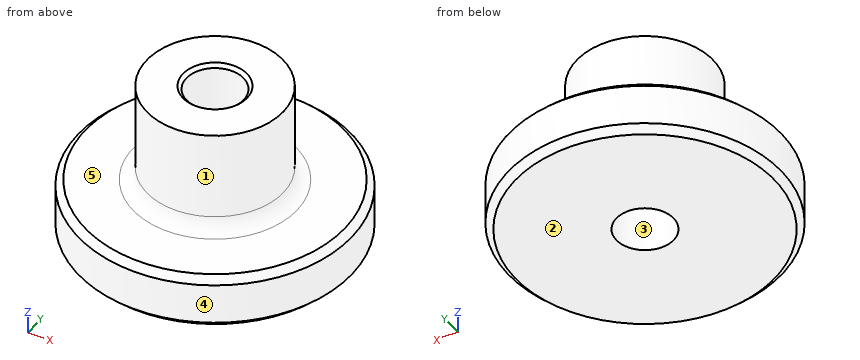
```python
from build123d import *

# Parameters (mm, degrees)
CROQUIS1_R              = 10
CROQUIS1_R_2            = 2.1
SALIENTE_EXTRUIR1_DEPTH = 4
CROQUIS2_R              = 5
CROQUIS2_R_2            = 2.1
SALIENTE_EXTRUIR2_DEPTH = 7.5
CHAFL_N1_SIZE           = 0.5
REDONDEO1_R             = 1
CHAFL_N2_SIZE           = 0.25


with BuildPart() as part:
    # Croquis1 → Saliente-Extruir1 (new body)
    with BuildSketch(Plane.XY):
        Circle(CROQUIS1_R)
        Circle(CROQUIS1_R_2, mode=Mode.SUBTRACT)
    extrude(amount=SALIENTE_EXTRUIR1_DEPTH)

    # Croquis2 → Saliente-Extruir2 (add)
    with BuildSketch(Plane.XY.offset(4)):
        Circle(CROQUIS2_R)
        Circle(CROQUIS2_R_2, mode=Mode.SUBTRACT)
    extrude(amount=SALIENTE_EXTRUIR2_DEPTH)

    # Chaflán1
    chafl_n1_edges = [part.edges().sort_by_distance(p)[0] for p in [
        (-10, 0, 0),
        (-10, 0, 4),
    ]]
    chamfer(chafl_n1_edges, length=CHAFL_N1_SIZE)

    # Redondeo1
    redondeo1_edges = [part.edges().sort_by_distance(p)[0] for p in [
        (-5, 0, 4),
    ]]
    fillet(redondeo1_edges, radius=REDONDEO1_R)

    # Chaflán2
    chafl_n2_edges = [part.edges().sort_by_distance(p)[0] for p in [
        (-2.1, 0, 11.5),
    ]]
    chamfer(chafl_n2_edges, length=CHAFL_N2_SIZE)


solid = part.part
```
Verification items for the finished model (mm, model axes). Face numbers are marked on the shaded views. A direction names the side the tool comes from. Give positions to 0.01 mm unless a question says otherwise; leave off trailing zeros. Order: outer loops, then holes, each group sorted by start corner. A loop starts at its lowest first (then second) coordinate and runs counter-clockwise, first axis right, second up. Notation, with made-up numbers: M 53,30.5 L 94,30.5 A19 ccw 94,66.5 Z; hole C 80.25,-28.75 d7. An arc over 180 degrees is marked long. Answer in a Markdown table with one row per item. Add a question column.
Item 1: Scan lines: probe 1 along Y at (x, z) = (0, 7.75); probe 2 along Y at (x, z) = (0, 3); probe 3 along Z at (x, y) = (2, -7.75). Record each from-to range of solid material in increasing order. Write a range as from..to.
Item 2: Mould release check, pull along X, two halves, no side actions. Record for the marked faces 3, 4 and 5: released by +X, released by -X, zero draft, split by the parting line, or undercut.
Item 3: Section check D-D, the plane z = 9.5. Enter the section's corners in (x, y).
Item 4: Gauge pin test, flat ends, axial feed: pin 1 (5 mm diameter, centred on x = -6, z = 8.5, fed in from +Y); pin 2 (3 mm diameter, centred on y = -2, z = 6.5, fed in from +X); pin 3 (2 mm diameter, centred on x = -2, z = 2, fed in from +Y). Record the tip position at first contact, or that the pin passes through.
Item 5: Section check C-C, the plane z = 2.75. Enter the section's corners in (x, y).
Item 6: Tool access check on the marked faces 1 and 2. Record the directions out of +Z, -Z, +X, -X, +Y, -Y that give a thin tool (end or side, any length) a straight path to the whole face; none if there is none.
Item 7: Section check A-A, the plane x = 0. Enter the section's corners in (y, z).
Filled sheet:
| question | item | result |
|---|---|---|
| 1 | probe 1 | y = -5..-2.1, 2.1..5 |
| 1 | probe 2 | y = -10..-2.1, 2.1..10 |
| 1 | probe 3 | z = 0..4 |
| 2 | face 3 | undercut |
| 2 | face 4 | split by the parting line |
| 2 | face 5 | zero draft |
| 3 | outline | C 0,0 d10; hole C 0,0 d4.2 |
| 4 | pin 1 | stops at y = 3.57 |
| 4 | pin 2 | stops at x = 4.97 |
| 4 | pin 3 | stops at y = 9.95 |
| 5 | outline | C 0,0 d20; hole C 0,0 d4.2 |
| 6 | face 1 | +Z |
| 6 | face 2 | -Z, +X, -X, +Y, -Y |
| 7 | outline | M -10,0.5 L -9.5,0 L -2.1,0 L -2.1,11.25 L -2.35,11.5 L -5,11.5 L -5,5 A1 cw -6,4 L -9.5,4 L -10,3.5 Z; M 2.1,0 L 9.5,0 L 10,0.5 L 10,3.5 L 9.5,4 L 6,4 A1 cw 5,5 L 5,11.5 L 2.35,11.5 L 2.1,11.25 Z |
